```python
from build123d import *

# Parameters (mm, degrees)
F1_DEPTH = 40.894


with BuildPart() as f1:
    # F0 (on Front) → F1 (new body)
    with BuildSketch(Plane.XZ):
        with BuildLine():
            Line((-26.524263, 21.714916), (-19.820329, 19.740981))
            Line((-19.820329, 19.740981), (-19.820329, 49.912829))
            ThreePointArc((-19.820329, 49.912829), (-20.013098, 50.378215), (-20.478483, 50.570983))
            Line((-20.478483, 50.570983), (-21.048689, 50.570983))
            ThreePointArc((-21.048689, 50.570983), (-25.538817, 48.711112), (-27.398689, 44.220983))
            Line((-27.398689, 44.220983), (-27.398689, 6.35))
            ThreePointArc((-27.398689, 6.35), (-25.538817, 1.859872), (-21.048689, 0))
            Line((-21.048689, 0), (0, 0))
            Line((0, 0), (12.430089, 0))
            Line((12.430089, 0), (12.430089, 4.517869))
            Line((12.430089, 4.517869), (0, 4.517869))
            Line((0, 4.517869), (-13.470329, 4.517869))
            ThreePointArc((-13.470329, 4.517869), (-17.960457, 6.377741), (-19.820329, 10.867869))
            Line((-19.820329, 10.867869), (-19.820329, 15.958715))
            Line((-19.820329, 15.958715), (-26.524263, 17.925737))
            Line((-26.524263, 17.925737), (-26.524263, 21.714916))
        make_face()
        Polygon((-19.820329, 15.958715), (-19.820329, 19.740981), (-26.524263, 21.714916), (-26.524263, 17.925737), align=None)
    extrude(amount=-F1_DEPTH)


solid = f1.part
```
Build history of the part. All positions in model axes, mm. A direction names the side the tool comes from. Round coordinates to 2 decimals unless told otherwise and drop trailing zeros. Write each loop counter-clockwise with the first axis right and the second up, starting at its lowest first coordinate (ties: lowest second). Pieces come first, ordered by that corner, then holes. Notation, with made-up numbers: (18.25, 29) -> (58.25, 29) arc R18 ccw to (58.25, 45) -> close; hole circle Ø7 at (-23, 52). An arc over 180 degrees is marked (long way). Put each result on its own line as item: value.
Item 1: Slice it at B-B, the plane z = 11.5. Give the cut face in (x, y), plus the area to 3 significant figures.
Here are the results:
outline: (-27.4, 0) -> (-19.82, 0) -> (-19.82, 40.89) -> (-27.4, 40.89) -> close
area: 310 mm^2
Item 2: Flat gauge pins, fed straight in: P1, Ø20.5, axis at x = -0.5, y = 28, coming from the +Z side; P2, Ø4, axis at y = 29, z = 24.5, coming from the +X side; P3, Ø3, axis at x = -3.5, y = 20.5, coming from the -Z side; P4, Ø3, axis at x = -16.5, z = 19, coming from the -Y side. Where does each tip first touch, or does it go through?
Here are the results:
P1: stops at z = 4.52
P2: stops at x = -19.82
P3: stops at z = 0
P4: passes through
Item 3: Wall check: probe 1 along X at (y, z) = (37, 37.5); probe 2 along Z at (x, y) = (-9, 9.5); probe 3 along X at (y, z) = (38.5, 8.5). Give the ranges that are in metal, low to high. Write a range as from..to.
Here are the results:
probe 1: x = -27.4..-19.82
probe 2: z = 0..4.52
probe 3: x = -27.4..-19.36
Item 4: Slice it at C-C, the plane x = 6.5. Give the cut face in (y, z), plus the area to 3 significant figures.
Here are the results:
outline: (0, 0) -> (40.89, 0) -> (40.89, 4.52) -> (0, 4.52) -> close
area: 185 mm^2
Item 5: Slice it at A-A, the plane y = 11.5. Give the cut face in (x, z), plus the area to 3 significant figures.
Here are the results:
outline: (-27.4, 6.35) arc R6.35 ccw to (-21.05, 0) -> (12.43, 0) -> (12.43, 4.52) -> (-13.47, 4.52) arc R6.35 cw to (-19.82, 10.87) -> (-19.82, 49.91) arc R0.66 ccw to (-20.48, 50.57) -> (-21.05, 50.57) arc R6.35 ccw to (-27.4, 44.22) -> close
area: 520 mm^2
Item 6: Tool access for faces 1 (the face through (-21, 0, 20)), 2 (the face through (0, 20, 4.518)): list every direction of +Z, -Z, +X, -X, +Y, -Y with a clear straight run to the whole face (end or side of a thin tool).
Here are the results:
face 1: +Z, -Z, +X, -X, -Y
face 2: +Z, +X, +Y, -Y
